The listing builds one solid part. Answer for the finished solid, in the listing's coordinates (mm). A direction names the side the tool comes from. Give positions to 0.01 mm unless a question says otherwise; leave off trailing zeros. Write each loop counter-clockwise with the first axis right and the second up, starting at its lowest first coordinate (ties: lowest second). Pieces come first, ordered by that corner, then holes.
```python
from build123d import *

# Parameters (mm, degrees)
BASPROSKE_W        = 5
BASPROSKE_H        = 22
TOOTHCUT_DEPTH     = 32.511902513
TEETHCUTS_COUNT    = 20
TEETHCUTS_ANGLE    = 342
BORSKE_R           = 0.5
BORE_DEPTH         = 50.0000508
SKETCH1_R          = 11.1
CUT_EXTRUDE1_DEPTH = 10


with BuildPart() as part:
    # BasProSke → Base-Revolve (revolve)
    with BuildSketch(Plane(origin=(0, 0, 0), x_dir=(1, 0, 0), z_dir=(0, 1, 0)), mode=Mode.PRIVATE) as base_revolve_sk:
        with Locations((2.5, 11)):
            Rectangle(BASPROSKE_W, BASPROSKE_H)
    revolve(base_revolve_sk.sketch.rotate(Axis((-10, 0, 0), (1, 0, 0)), 180), axis=Axis((-10, 0, 0), (1, 0, 0)))

    # TooCutSke → ToothCut (cut, through all)
    with BuildSketch(Plane(origin=(0, 0, 0), x_dir=(0, 0, -1), z_dir=(1, 0, 0))):
        with BuildLine():
            ThreePointArc((0.986171591, 17.471189616), (0, 17.499), (-0.986171591, 17.471189616))
            ThreePointArc((-0.986171591, 17.471189616), (-1.626916196, 19.798789858), (-2.932850173, 21.829260982))
            ThreePointArc((-2.932850173, 21.829260982), (0, 22.0254), (2.932850173, 21.829260982))
            ThreePointArc((2.932850173, 21.829260982), (1.626916196, 19.798789858), (0.986171591, 17.471189616))
        make_face()
    toothcut = extrude(amount=TOOTHCUT_DEPTH, mode=Mode.SUBTRACT)

    # TeethCuts: ToothCut ×20 about axis
    teethcuts_axis = Axis((-10, 0, 0), (1, 0, 0))
    for i in range(1, TEETHCUTS_COUNT):
        add(toothcut.rotate(teethcuts_axis, i * TEETHCUTS_ANGLE / (TEETHCUTS_COUNT - 1)), mode=Mode.SUBTRACT)

    # BorSke → Bore (cut, symmetric)
    with BuildSketch(Plane(origin=(0, 0, 0), x_dir=(0, 0, -1), z_dir=(1, 0, 0))):
        with Locations(Location((0, 0, 0), (0, 0, 180))):
            Circle(BORSKE_R)
    extrude(amount=BORE_DEPTH, both=True, mode=Mode.SUBTRACT)

    # Sketch1 → Cut-Extrude1 (cut)
    with BuildSketch(Plane.ZY):
        Circle(SKETCH1_R)
    extrude(amount=-CUT_EXTRUDE1_DEPTH, mode=Mode.SUBTRACT)


solid = part.part
```
Item 1: Consider probe 1 along Z at (x, y) = (4.5, -19); probe 2 along Z at (x, y) = (3.5, -17); probe 3 along Y at (x, z) = (4.45, 15). Determine where each line is inside the solid, lowest interval first.
Conclusion:
probe 1: z = -10.49 to -8.35, -4.6 to -1.32, 1.32 to 4.6, 8.35 to 10.49
probe 2: z = -10.33 to -6.7, -4.48 to 4.48, 6.7 to 10.33
probe 3: y = -15.89 to -12.85, -9.62 to 9.62, 12.85 to 15.89
Item 2: A cutting plane is placed at C-C, the plane z = -12.5. Give the vertices of the cut face in (x, y).
Conclusion:
outline: (0, -14.78) - (5, -14.78) - (5, 14.78) - (0, 14.78) - close
Item 3: Each of these flat-tipped pins is pushed along its axis until it touches: P1, Ø2, axis at x = 1.5, z = 12.5, coming from the -Y side; P2, Ø1.5, axis at x = 3.5, y = 2.5, coming from the +Z side; P3, Ø1, axis at x = 1.5, y = 12.5, coming from the +Z side. Where does it stop, or does it pass through?
Conclusion:
P1: stops at y = -15.35
P2: stops at z = 21.81
P3: stops at z = 15.09
Item 4: Which of the six approach directions +Z, -Z, +X, -X, +Y, -Y give full straight-line access (tool end or side, diameter ignored) to faces 1 (the face through (2.54, -9.99, -19.6)), 2 (the face through (2.535, 3.449, 21.728)), 3 (the face through (2.465, -15.037, -12.911)), 4 (the face through (2.46, 10.31, 16.93)), 5 (the face through (2.465, -12.911, 15.037))?
Conclusion:
face 1: -Z, +X, -X, -Y
face 2: +Z, +X, -X, +Y
face 3: +X, -X, -Y
face 4: +X, -X
face 5: +Z, +X, -X
Item 5: A cutting plane is placed at A-A, the plane z = 0. Give the vertices of the cut face in (x, y).
Conclusion:
outline: (0, -17.5) - (5, -17.5) - (5, -11.1) - (0, -11.1) - close; (0, 11.1) - (5, 11.1) - (5, 17.5) - (0, 17.5) - close
Item 6: A cutting plane is placed at D-D, the plane y = 12. Give the vertices of the cut face in (x, z).
Conclusion:
outline: (0, -14.42) - (5, -14.42) - (5, 14.42) - (0, 14.42) - close
Item 7: Determine the mould class of faces 6 (the face through (2.54, 3.43, -21.73)), 7 (the face through (2.465, 14.149, -10.297)), 8 (the face through (2.54, 21.73, 3.43)) for opening direction Z: pulls with the +Z half, pulls with the -Z half, needs draft (parallel to the pull), parting line crosses it, or undercut.
Conclusion:
face 6: pulls with the -Z half
face 7: undercut
face 8: pulls with the +Z half
